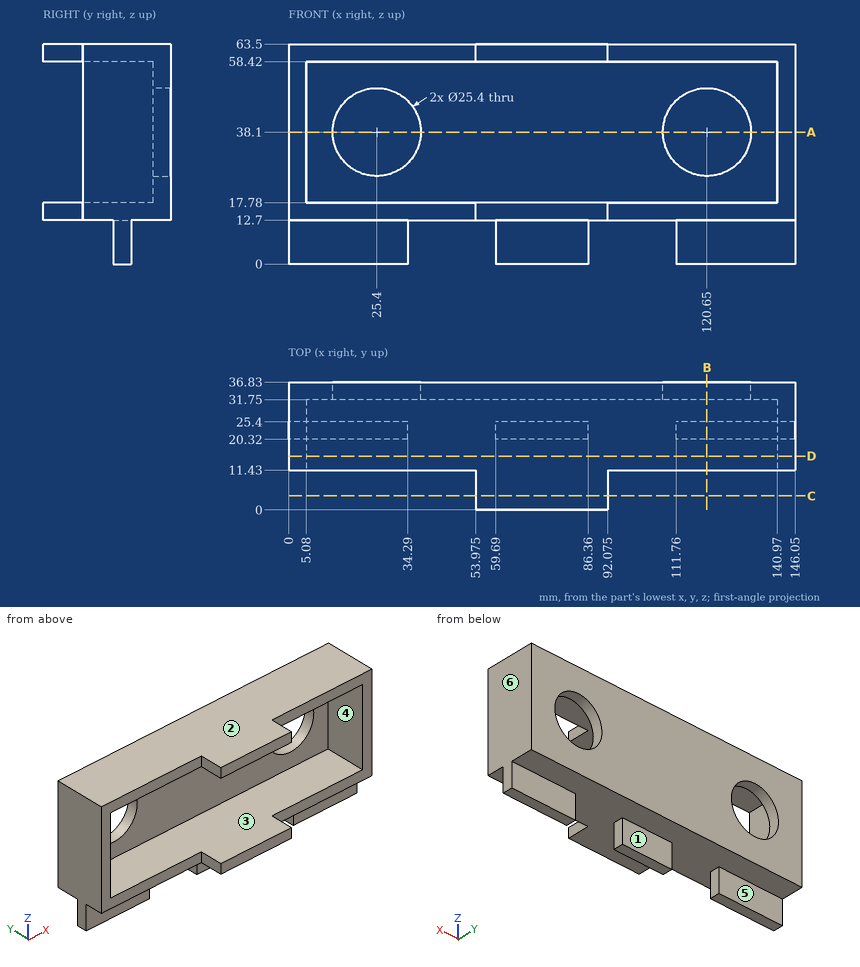
Can you work these out from the drawing? Everything is in mm from the part's minimum corner. A direction names the side the tool comes from. Coordinates: 2 decimals unless noted, no trailing zeros. Loops run counter-clockwise (first coordinate to the right, second up) from the corner with the lowest first, then second, coordinate; pieces in that order, holes last. Notation, with made-up numbers: (-15, -8) - (18, -8) arc R32 ccw to (18, 18) - close; hole circle Ø8 at (-31.75, 15). An arc over 180 degrees is marked (long way). Use a Markdown table: item, result.
Item 1: Will these pins go through, and if not, where does the flat tip stop? pin 1 (4 mm diameter, centred on x = 15.5, z = 9, fed in from +Y); pin 2 (2.5 mm diameter, centred on y = 6, z = 15.5, fed in from +X) (3 decimals); pin 3 (5.5 mm diameter, centred on y = 3, z = 15, fed in from -X) (3 decimals).
Numbers:
| item | result |
|---|---|
| pin 1 | stops at y = 25.4 |
| pin 2 | stops at x = 92.075 |
| pin 3 | stops at x = 53.975 |
Item 2: I want a section at C-C on y = 4. Please give me the cut outline in (x, z) (3 decimals), and give its area (3 significant figures).
Numbers:
| item | result |
|---|---|
| outline | (53.975, 12.7) - (92.075, 12.7) - (92.075, 17.78) - (53.975, 17.78) - close; (53.975, 58.42) - (92.075, 58.42) - (92.075, 63.5) - (53.975, 63.5) - close |
| area | 387 mm2 |
Item 3: I want a section at D-D on y = 15.5. Please give me the cut outline in (x, z), and give its area (3 significant figures).
Numbers:
| item | result |
|---|---|
| outline | (0, 12.7) - (146.05, 12.7) - (146.05, 63.5) - (0, 63.5) - close; hole (5.08, 17.78) - (140.97, 17.78) - (140.97, 58.42) - (5.08, 58.42) - close |
| area | 1,900 mm2 |
Item 4: We'd pull the mould along Z, two halves only. Please class the marked faces 1, 2 and 3: released by +Z, released by -Z, zero draft, split by the parting line, or undercut.
Numbers:
| item | result |
|---|---|
| face 1 | zero draft |
| face 2 | released by +Z |
| face 3 | undercut |
Item 5: I want a section at B-B on x = 120.65. Please give me the cut outline in (y, z), and give its area (3 significant figures).
Numbers:
| item | result |
|---|---|
| outline | (11.43, 12.7) - (20.32, 12.7) - (20.32, 0) - (25.4, 0) - (25.4, 12.7) - (36.83, 12.7) - (36.83, 25.4) - (31.75, 25.4) - (31.75, 17.78) - (11.43, 17.78) - close; (11.43, 58.42) - (31.75, 58.42) - (31.75, 50.8) - (36.83, 50.8) - (36.83, 63.5) - (11.43, 63.5) - close |
| area | 400 mm2 |
Item 6: For the marked faces 4, 5 and 6, which set-ups out of +Z, -Z, +X, -X, +Y, -Y let a thin tool reach every point of the face, with its end or its side?
Numbers:
| item | result |
|---|---|
| face 4 | -Y |
| face 5 | -Z, +X, -X, +Y |
| face 6 | +Z, -Z, +X, +Y, -Y |
Item 7: I want a section at A-A on z = 38.1. Please give me the cut outline in (x, y), and give its area (3 significant figures).
Numbers:
| item | result |
|---|---|
| outline | (0, 11.43) - (5.08, 11.43) - (5.08, 31.75) - (12.7, 31.75) - (12.7, 36.83) - (0, 36.83) - close; (38.1, 31.75) - (107.95, 31.75) - (107.95, 36.83) - (38.1, 36.83) - close; (133.35, 31.75) - (140.97, 31.75) - (140.97, 11.43) - (146.05, 11.43) - (146.05, 36.83) - (133.35, 36.83) - close |
| area | 690 mm2 |
Item 8: If I drill on probe 1 along X at (y, z) = (23, 10); probe 2 along X at (y, z) = (35, 38.1); probe 3 along Z at (x, y) = (10, 25), over which ranges is the centre line in solid material (lowest first)? Write a range as from..to.
Numbers:
| item | result |
|---|---|
| probe 1 | x = 0..34.29, 59.69..86.36, 111.76..146.05 |
| probe 2 | x = 0..12.7, 38.1..107.95, 133.35..146.05 |
| probe 3 | z = 0..17.78, 58.42..63.5 |
